Here's how the part is built. I have some questions about the finished solid (model axes, mm). Face numbers are marked on the shaded views. A direction names the side the tool comes from. Round coordinates to 2 decimals unless told otherwise and drop trailing zeros. Loops run counter-clockwise (first coordinate to the right, second up) from the corner with the lowest first, then second, coordinate; pieces in that order, holes last. Notation, with made-up numbers: (55, -25.5) -> (103, -25.5) arc R28 ccw to (103, -5.5) -> close; hole circle Ø3 at (13, -10). An arc over 180 degrees is marked (long way). Use one line per item in the form item = value. Start each with the question number.
Item 1: If we section it at C-C (z = 2): Write out the boundary of the cut face in (x, y), then the cut area to 3 significant figures.
Item 2: Thinking about a two-plate mould opening in Z: for the marked faces 1, 2, 3 and 4, which applies, released by +Z, released by -Z, zero draft, split by the parting line, or undercut?
Item 3: If I drill on L1, parallel to Z at x = -2.75, y = 19; L2, parallel to X at y = 16, z = -0.5; L3, parallel to Y at x = 11.75, z = 3, over which ranges is the centre line in solid material (lowest first)? Write a range as [from, to].
Item 4: If we section it at D-D (y = 40): Write out the boundary of the cut face in (x, z), then the cut area to 3 significant figures.
Item 5: If we section it at B-B (y = 34): Write out the boundary of the cut face in (x, z).
Item 6: For the marked faces 5, 6, 7, 8 and 9, which set-ups out of +Z, -Z, +X, -X, +Y, -Y let a thin tool reach every point of the face, with its end or its side?
Item 7: I'm going to push a flat-ended pin straight in: pin 1 Ø1.5 at (y, z) = (53, 5.5) entering from -X. Where does the tip first touch, or does it pass through?
Item 8: If we section it at A-A (x = -3.5): Write out the boundary of the cut face in (y, z), then the cut area to 3 significant figures.
```python
from build123d import *

# Parameters (mm, degrees)
SKETCH_1_W          = 30
SKETCH_1_H          = 30
EXTRUDE_2_DEPTH     = 60
SKETCH_2_W          = 22
SKETCH_2_H          = 10
CUT_EXTRUDE_1_DEPTH = 47
SKETCH_3_W          = 17
SKETCH_3_H          = 12
CUT_EXTRUDE_2_DEPTH = 31
SKETCH_5_W          = 17
SKETCH_5_H          = 17
CUT_EXTRUDE_3_DEPTH = 5
SKETCH_6_W          = 12
SKETCH_6_H          = 17
CUT_EXTRUDE_4_DEPTH = 31
SKETCH_7_W          = 17
SKETCH_7_H          = 17
CUT_EXTRUDE_5_DEPTH = 5
FILLET_1_R          = 1
FILLET_2_R          = 1
FILLET_3_R          = 1
FILLET_4_R          = 1
FILLET_5_R          = 1


with BuildPart() as part:
    # ｽｹｯﾁ1 → ﾎﾞｽ - 押し出し2 (new body)
    with BuildSketch(Plane(origin=(0, 0, 0), x_dir=(1, 0, 0), z_dir=(0, 1, 0))):
        Rectangle(SKETCH_1_W, SKETCH_1_H)
    extrude(amount=EXTRUDE_2_DEPTH)

    # ｽｹｯﾁ2 → ｶｯﾄ - 押し出し1 (cut)
    with BuildSketch(Plane.XZ):
        Rectangle(SKETCH_2_W, SKETCH_2_H)
    extrude(amount=-CUT_EXTRUDE_1_DEPTH, mode=Mode.SUBTRACT)

    # ｽｹｯﾁ3 → ｶｯﾄ - 押し出し2 (cut, through all)
    with BuildSketch(Plane(origin=(15, 0, 0), x_dir=(0, 0, -1), z_dir=(1, 0, 0))):
        with Locations((0, 49)):
            Rectangle(SKETCH_3_W, SKETCH_3_H)
    extrude(amount=-CUT_EXTRUDE_2_DEPTH, mode=Mode.SUBTRACT)

    # ｽｹｯﾁ5 → ｶｯﾄ - 押し出し3 (cut)
    with BuildSketch(Plane(origin=(0, 60, 0), x_dir=(1, 0, 0), z_dir=(0, 1, 0))):
        Rectangle(SKETCH_5_W, SKETCH_5_H)
    extrude(amount=-CUT_EXTRUDE_3_DEPTH, mode=Mode.SUBTRACT)

    # ｽｹｯﾁ6 → ｶｯﾄ - 押し出し4 (cut, through all)
    with BuildSketch(Plane(origin=(15, 0, 0), x_dir=(0, 0, -1), z_dir=(1, 0, 0))):
        with Locations((-4, 29.5)):
            Rectangle(SKETCH_6_W, SKETCH_6_H)
    extrude(amount=-CUT_EXTRUDE_4_DEPTH, mode=Mode.SUBTRACT)

    # ｽｹｯﾁ7 → ｶｯﾄ - 押し出し5 (cut)
    with BuildSketch(Plane.XY.offset(15)):
        with Locations((0, 29.5)):
            Rectangle(SKETCH_7_W, SKETCH_7_H)
    extrude(amount=-CUT_EXTRUDE_5_DEPTH, mode=Mode.SUBTRACT)

    # ﾌｨﾚｯﾄ1
    fillet_1_edges = [part.edges().sort_by_distance(p)[0] for p in [
        (15, 30, 15),
    ]]
    fillet(fillet_1_edges, radius=FILLET_1_R)

    # ﾌｨﾚｯﾄ2
    fillet_2_edges = [part.edges().sort_by_distance(p)[0] for p in [
        (15, 0, -0.5),
        (14.707106781, 0, 14.707106781),
        (-0.5, 0, 15),
    ]]
    fillet(fillet_2_edges, radius=FILLET_2_R)

    # ﾌｨﾚｯﾄ3
    fillet_3_edges = [part.edges().sort_by_distance(p)[0] for p in [
        (-0.5, 0, -15),
        (14.707106781, 0.292893219, -15),
        (15, 30.5, -15),
    ]]
    fillet(fillet_3_edges, radius=FILLET_3_R)

    # ﾌｨﾚｯﾄ4
    fillet_4_edges = [part.edges().sort_by_distance(p)[0] for p in [
        (15, 60, 0),
        (14.707106781, 60, 14.707106781),
        (-0.5, 60, -15),
        (14.707106781, 60, -14.707106781),
        (-0.5, 60, 15),
    ]]
    fillet(fillet_4_edges, radius=FILLET_4_R)

    # ﾌｨﾚｯﾄ5
    fillet_5_edges = [part.edges().sort_by_distance(p)[0] for p in [
        (-15, 0.292893219, 14.707106781),
        (-15, 0, 0),
        (-15, 0.292893219, -14.707106781),
        (-15, 60, 0),
        (-15, 30, 15),
        (-15, 30, -15),
        (-15, 59.707106781, -14.707106781),
        (-15, 59.707106781, 14.707106781),
    ]]
    fillet(fillet_5_edges, radius=FILLET_5_R)


solid = part.part
```
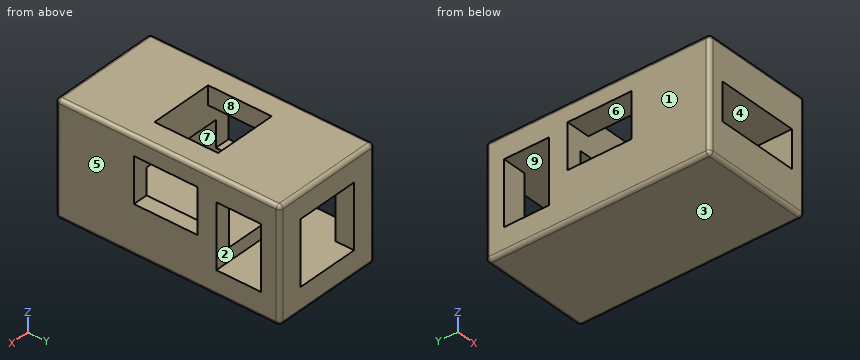
Values found:
q1.outline = (-15, 1) arc R1 ccw to (-14, 0) -> (-11, 0) -> (-11, 21) -> (-15, 21) -> close; (-15, 38) -> (-11, 38) -> (-11, 43) -> (-15, 43) -> close; (-15, 55) -> (-8.5, 55) -> (-8.5, 60) -> (-14, 60) arc R1 ccw to (-15, 59) -> close; (8.5, 55) -> (15, 55) -> (15, 59) arc R1 ccw to (14, 60) -> (8.5, 60) -> close; (11, 0) -> (14, 0) arc R1 ccw to (15, 1) -> (15, 21) -> (11, 21) -> close; (11, 38) -> (15, 38) -> (15, 43) -> (11, 43) -> close
q1.area = 272 mm2
q2.face_1 = zero draft
q2.face_2 = undercut
q2.face_3 = released by -Z
q2.face_4 = undercut
q3.L1 = [-15, -5], [5, 15]
q3.L2 = [-15, -11], [11, 15]
q3.L3 = [0, 21], [38, 43], [55, 60]
q4.outline = (-15, -14) arc R1 ccw to (-14, -15) -> (14, -15) arc R1 ccw to (15, -14) -> (15, 14) arc R1 ccw to (14, 15) -> (-14, 15) arc R1 ccw to (-15, 14) -> close; hole (-11, -5) -> (11, -5) -> (11, 5) -> (-11, 5) -> close
q4.area = 679 mm2
q5.outline = (-15, -14) arc R1 ccw to (-14, -15) -> (14, -15) arc R1 ccw to (15, -14) -> (15, -2) -> (11, -2) -> (11, -5) -> (-11, -5) -> (-11, -2) -> (-15, -2) -> close; (-15, 10) -> (-8.5, 10) -> (-8.5, 15) -> (-14, 15) arc R1 ccw to (-15, 14) -> close; (8.5, 10) -> (15, 10) -> (15, 14) arc R1 ccw to (14, 15) -> (8.5, 15) -> close
q6.face_5 = +Z, -Z, +X, +Y, -Y
q6.face_6 = +X, -X
q6.face_7 = -Y
q6.face_8 = +Z
q6.face_9 = none
q7.pin_1 = through
q8.outline = (0, -14) arc R1 ccw to (1, -15) -> (59, -15) arc R1 ccw to (60, -14) -> (60, -8.5) -> (43, -8.5) -> (43, -5) -> (0, -5) -> close; (0, 5) -> (21, 5) -> (21, 15) -> (1, 15) arc R1 ccw to (0, 14) -> close; (38, 5) -> (43, 5) -> (43, 8.5) -> (60, 8.5) -> (60, 14) arc R1 ccw to (59, 15) -> (38, 15) -> close
q8.area = 910 mm2
